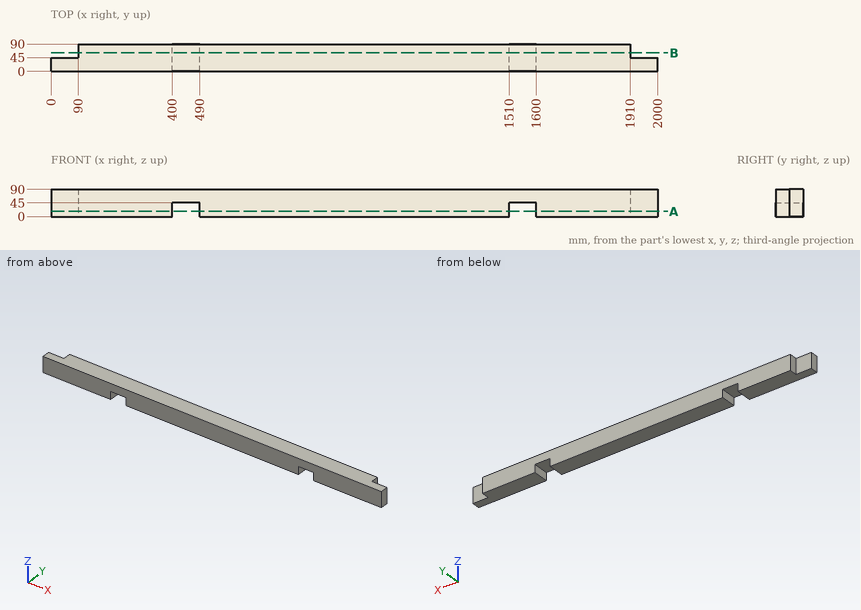
The figure shows three views and two pictorial views of one solid part (mm, origin at its lowest corner). Answer the questions. Coordinates: 2 decimals unless noted, no trailing zeros. Loops run counter-clockwise (first coordinate to the right, second up) from the corner with the lowest first, then second, coordinate; pieces in that order, holes last. Notation, with made-up numbers: (30, 42.25) - (60, 42.25) arc R14 ccw to (60, 60.25) - close; hole circle Ø11 at (54.25, 6). An arc over 180 degrees is marked (long way). Use a Markdown table: item, result. Add a question column.
1) The part is cut by section B-B, the plane y = 60.5. Give the vertices of the cut face in (x, z), and give its area (3 significant figures).
2) Find the intervals of material crossed by line 1 (X direction, y = 80.5, z = 9); line 2 (X direction, y = 30.5, z = 19.5); line 3 (X direction, y = 57.5, z = 54), in increasing order.
3) Given pin 1 (22.5 mm diameter, centred on y = 61, z = 31, fed in from +X); pin 2 (13.5 mm diameter, centred on y = 52, z = 30.5, fed in from -X), each flat-ended and moving along its own axis, determine where each tip first touches the part or whether it passes through.
4) The part is cut by section A-A, the plane z = 17. Give the vertices of the cut face in (x, y), and give its area (3 significant figures).
Here are the results:
| question | item | result |
|---|---|---|
| 1 | outline | (90, 0) - (400, 0) - (400, 45) - (490, 45) - (490, 0) - (1510, 0) - (1510, 45) - (1600, 45) - (1600, 0) - (1910, 0) - (1910, 90) - (90, 90) - close |
| 1 | area | 156,000 mm^2 |
| 2 | line 1 | x = 90 to 400, 490 to 1510, 1600 to 1910 |
| 2 | line 2 | x = 0 to 400, 490 to 1510, 1600 to 2000 |
| 2 | line 3 | x = 90 to 1910 |
| 3 | pin 1 | stops at x = 1910 |
| 3 | pin 2 | stops at x = 90 |
| 4 | outline | (0, 0) - (400, 0) - (400, 90) - (90, 90) - (90, 45) - (0, 45) - close; (490, 0) - (1510, 0) - (1510, 90) - (490, 90) - close; (1600, 0) - (2000, 0) - (2000, 45) - (1910, 45) - (1910, 90) - (1600, 90) - close |
| 4 | area | 156,000 mm^2 |
